from build123d import *

# Parameters (mm, degrees)
SKETCH1_R              = 13.768224287
SKETCH1_R_2            = 12.268224287
SKETCH1_R_3            = 10.768224287
BOSS_EXTRUDE1_DEPTH    = 6.5
CUT_EXTRUDE3_DEPTH     = 519.353793234
CUT_EXTRUDE1_START     = -1.3
CUT_EXTRUDE1_DEPTH     = 13
CUT_EXTRUDE8_START     = -1.75
CUT_EXTRUDE8_OUTLINE_R = 10.768224287
CUT_EXTRUDE8_DEPTH     = 1.75
SKETCH6_R              = 12.268224287
CUT_EXTRUDE9_DEPTH     = 1.3
CUT_EXTRUDE12_START    = -1.75
CUT_EXTRUDE12_DEPTH    = 1.75
SKETCH8_R              = 2.5
CUT_EXTRUDE13_DEPTH    = 63.803249571
CHAMFER1_SIZE          = 2.5
CUT_EXTRUDE14_START    = -3.45
CUT_EXTRUDE14_DEPTH    = 3.45


# Read off the part's stored shape, not the designer's step: Cut-Extrude8
with BuildPart() as part:
    # Sketch1 → Boss-Extrude1 (new, symmetric)
    # profile 1 of 6: a face of its own
    with BuildSketch(Plane(origin=(0, 0, 0), x_dir=(0, 0, -1), z_dir=(1, 0, 0))):
        with BuildLine():
            Line((0, 5), (0, 0))
            Line((0, 0), (15, 0))
            Line((15, 0), (15, 0.231775713))
            Line((15, 0.231775713), (15.418491318, 8.357342638))
            ThreePointArc((15.418491318, 8.357342638), (14.445072398, 11.461887277), (14.227329557, 14.708166664))
            Line((14.227329557, 14.708166664), (13.727329557, 5))
            Line((13.727329557, 5), (0, 5))
        make_face()
    # profile 2 of 6: a face of its own
    with BuildSketch(Plane(origin=(0, 0, 0), x_dir=(0, 0, -1), z_dir=(1, 0, 0))):
        with BuildLine():
            Line((15.418491318, 8.357342638), (15, 0.231775713))
            Line((15, 0.231775713), (27.977329557, 0.231775713))
            ThreePointArc((27.977329557, 0.231775713), (20.498204345, 2.440299049), (15.418491318, 8.357342638))
        make_face()
    # profile 3 of 6: a face of its own
    with BuildSketch(Plane(origin=(0, 0, 0), x_dir=(0, 0, -1), z_dir=(1, 0, 0))):
        with BuildLine():
            ThreePointArc((40.536167797, 8.357342638), (35.45645477, 2.440299049), (27.977329557, 0.231775713))
            Line((27.977329557, 0.231775713), (40.954659115, 0.231775713))
            Line((40.954659115, 0.231775713), (40.536167797, 8.357342638))
        make_face()
    # profile 4 of 6: a face of its own
    with BuildSketch(Plane(origin=(0, 0, 0), x_dir=(0, 0, -1), z_dir=(1, 0, 0))):
        with BuildLine():
            Line((42.227329557, 5), (41.727329557, 14.708166664))
            ThreePointArc((41.727329557, 14.708166664), (41.740997019, 14.354200561), (41.745553845, 14))
            ThreePointArc((41.745553845, 14), (41.439812643, 11.114597224), (40.536167797, 8.357342638))
            Line((40.536167797, 8.357342638), (40.954659115, 0.231775713))
            Line((40.954659115, 0.231775713), (40.954659115, 0))
            Line((40.954659115, 0), (55.954659115, 0))
            Line((55.954659115, 0), (55.954659115, 5))
            Line((55.954659115, 5), (42.227329557, 5))
        make_face()
    # profile 5 of 6: a face of its own
    with BuildSketch(Plane(origin=(0, 0, 0), x_dir=(0, 0, -1), z_dir=(1, 0, 0))):
        with Locations((27.977329557, 14)):
            Circle(SKETCH1_R)
        with Locations((27.977329557, 14)):
            Circle(SKETCH1_R_2, mode=Mode.SUBTRACT)
    # profile 6 of 6: a face of its own
    with BuildSketch(Plane(origin=(0, 0, 0), x_dir=(0, 0, -1), z_dir=(1, 0, 0))):
        with Locations((27.977329557, 14)):
            Circle(SKETCH1_R_2)
        with Locations(Location((27.977329557, 14, 0), (0, 0, 180))):
            Circle(SKETCH1_R_3, mode=Mode.SUBTRACT)
    extrude(amount=BOSS_EXTRUDE1_DEPTH, both=True)

    # Sketch3 → Cut-Extrude3 (cut, through all)
    with BuildSketch(Plane(origin=(0, -487.515659686, 0), x_dir=(-1, 0, 0), z_dir=(0, 0, 1))):
        Polygon((-4.75, -502.22382635), (-6.5, -492.515659686), (-6.5, -515.283883974), (-4.75, -515.283883974), align=None)
        Polygon((6.5, -515.283883974), (6.5, -492.515659686), (4.75, -502.22382635), (4.75, -515.283883974), align=None)
    extrude(amount=-CUT_EXTRUDE3_DEPTH, mode=Mode.SUBTRACT)

    # Sketch2 → Cut-Extrude1 (cut)
    with BuildSketch(Plane(origin=(0, 0, 0), x_dir=(0, 0, -1), z_dir=(1, 0, 0)).offset(CUT_EXTRUDE1_START)):
        with BuildLine():
            Line((15, 0.231775713), (27.977329557, 0.231775713))
            ThreePointArc((27.977329557, 0.231775713), (20.498204345, 2.440299049), (15.418491318, 8.357342638))
            Line((15.418491318, 8.357342638), (15, 0.231775713))
        make_face()
        with BuildLine():
            Line((27.977329557, 0.231775713), (40.954659115, 0.231775713))
            Line((40.954659115, 0.231775713), (40.536167797, 8.357342638))
            ThreePointArc((40.536167797, 8.357342638), (35.45645477, 2.440299049), (27.977329557, 0.231775713))
        make_face()
    cut_extrude1 = extrude(amount=-CUT_EXTRUDE1_DEPTH, mode=Mode.SUBTRACT)

    # Cut-Extrude8 outline → Cut-Extrude8 (cut)
    with BuildSketch(Plane.ZY.offset(6.5).offset(CUT_EXTRUDE8_START)):
        with BuildLine():
            Line((-40.225097809, 14.708166664), (-40.536167797, 8.357342638))
            ThreePointArc((-40.536167797, 8.357342638), (-27.977329557, 0.231775713), (-15.418491318, 8.357342638))
            Line((-15.418491318, 8.357342638), (-15.729561306, 14.708166664))
            ThreePointArc((-15.729561306, 14.708166664), (-27.977329557, 26.268224287), (-40.225097809, 14.708166664))
        make_face()
        with Locations((-27.977329557, 14)):
            Circle(CUT_EXTRUDE8_OUTLINE_R, mode=Mode.SUBTRACT)
    extrude(amount=CUT_EXTRUDE8_DEPTH, mode=Mode.SUBTRACT)

    # Sketch6 → Cut-Extrude9 (cut)
    with BuildSketch(Plane.ZY.offset(4.75)):
        with Locations(Location((-27.977329557, 14, 0), (0, 0, 270))):
            Circle(SKETCH6_R)
    cut_extrude9 = extrude(amount=-CUT_EXTRUDE9_DEPTH, mode=Mode.SUBTRACT)

    # Mirror2: Cut-Extrude1, Cut-Extrude9 across plane
    add(cut_extrude1.mirror(Plane(origin=(0, 0, 0), x_dir=(0, 0, 1), z_dir=(1, 0, 0))), mode=Mode.SUBTRACT)
    add(cut_extrude9.mirror(Plane(origin=(0, 0, 0), x_dir=(0, 0, 1), z_dir=(1, 0, 0))), mode=Mode.SUBTRACT)

    # Sketch7 → Cut-Extrude12 (cut)
    with BuildSketch(Plane(origin=(6.5, 0, 0), x_dir=(0, 0, -1), z_dir=(1, 0, 0)).offset(CUT_EXTRUDE12_START)):
        with BuildLine():
            ThreePointArc((38.396734532, 5), (39.588438578, 6.600936051), (40.536167797, 8.357342638))
            Line((40.536167797, 8.357342638), (40.225097809, 14.708166664))
            ThreePointArc((40.225097809, 14.708166664), (27.977329557, 26.268224287), (15.729561306, 14.708166664))
            Line((15.729561306, 14.708166664), (15.418491318, 8.357342638))
            ThreePointArc((15.418491318, 8.357342638), (16.366220536, 6.600936051), (17.557924583, 5))
            Line((17.557924583, 5), (22.065083427, 5))
            ThreePointArc((22.065083427, 5), (27.977329557, 3.231775713), (33.889575687, 5))
            Line((33.889575687, 5), (38.396734532, 5))
        make_face()
        with BuildLine():
            Line((22.065083427, 5), (17.557924583, 5))
            ThreePointArc((17.557924583, 5), (27.977329557, 0.231775713), (38.396734532, 5))
            Line((38.396734532, 5), (33.889575687, 5))
            ThreePointArc((33.889575687, 5), (27.977329557, 3.231775713), (22.065083427, 5))
        make_face()
    extrude(amount=CUT_EXTRUDE12_DEPTH, mode=Mode.SUBTRACT)

    # Sketch8 → Cut-Extrude13 (cut, through all)
    with BuildSketch(Plane.XZ):
        with Locations(Location((0, -48.977329557, 0), (0, 0, 270))):
            Circle(SKETCH8_R)
        with Locations(Location((0, -6.977329557, 0), (0, 0, 270))):
            Circle(SKETCH8_R)
    extrude(amount=-CUT_EXTRUDE13_DEPTH, mode=Mode.SUBTRACT)

    # Chamfer1
    chamfer1_edges = [part.edges().sort_by_distance(p)[0] for p in [
        (-6.5, 2.5, 0),
        (6.5, 2.5, -55.954659115),
        (-6.5, 2.5, -55.954659115),
        (6.5, 2.5, 0),
    ]]
    chamfer(chamfer1_edges, length=CHAMFER1_SIZE)

    # Sketch9 → Cut-Extrude14 (cut)
    with BuildSketch(Plane.ZY.offset(3.45).offset(CUT_EXTRUDE14_START)):
        with BuildLine():
            Line((-38.451328521, 16.5), (-39.988129995, 16.5))
            ThreePointArc((-39.988129995, 16.5), (-40.245553845, 14), (-39.988129995, 11.5))
            Line((-39.988129995, 11.5), (-38.451328521, 11.5))
            ThreePointArc((-38.451328521, 11.5), (-38.745553845, 14), (-38.451328521, 16.5))
        make_face()
        with BuildLine():
            ThreePointArc((-15.70910527, 14), (-15.773630921, 15.256609231), (-15.966529119, 16.5))
            Line((-15.966529119, 16.5), (-17.503330593, 16.5))
            ThreePointArc((-17.503330593, 16.5), (-17.282914559, 15.258627083), (-17.20910527, 14))
            ThreePointArc((-17.20910527, 14), (-17.282914559, 12.741372917), (-17.503330593, 11.5))
            Line((-17.503330593, 11.5), (-15.966529119, 11.5))
            ThreePointArc((-15.966529119, 11.5), (-15.773630921, 12.743390769), (-15.70910527, 14))
        make_face()
    extrude(amount=CUT_EXTRUDE14_DEPTH, mode=Mode.SUBTRACT)


solid = part.part
The listing builds one solid part. Answer for the finished solid, in the listing's coordinates (mm). A direction names the side the tool comes from. Round coordinates to 2 decimals unless told otherwise and drop trailing zeros. Write each loop counter-clockwise with the first axis right and the second up, starting at its lowest first coordinate (ties: lowest second). Pieces come first, ordered by that corner, then holes. Notation, with made-up numbers: M 26.25,29 L 46.25,29 A32 cw 46.25,57 Z; hole C 39,-6 d2. An arc over 180 degrees is marked long. Write each question's results on one line, items separated by ' | '. Start each with the question number.
Item 1: Find section A-A on z = -35. Write down the section's boundary in (x, y).
Item 2: The mould has two halves that part along Y. Classify faces 4 (the flat face through (-2, 16.5, -17)), 5 (the flat face through (6.5, 3, -9)), 6 (the flat face through (-5.06, 10.166, -40.448)): +Y half, -Y half, draft (parallel to the pull), parting line (faces both ways), or undercut.
Item 3: Find section C-C on z = -12. Write down the section's boundary in (x, y).
Item 4: Given pin 1 Ø2 at (x, z) = (2, -39.5) entering from -Y; pin 2 Ø4.5 at (y, z) = (4, -31) entering from -X; pin 3 Ø1.7 at (x, z) = (-2.5, -39) entering from +Y, each flat-ended and moving along its own axis, determine where each tip first touches the part or whether it passes through.
Item 5: Straight lines are drawn through the part: probe 1 along X at (y, z) = (2.75, -31); probe 2 along Y at (x, z) = (0.25, -46); probe 3 along X at (y, z) = (5, -17.5). For each, find the intervals that lie inside material, in ascending order.
Item 6: Which of the six approach directions +Z, -Z, +X, -X, +Y, -Y give full straight-line access (tool end or side, diameter ignored) to faces 1 (the flat face through (-5.187, 10.783, -15.537)), 2 (the flat face through (0, 0.232, -28)), 3 (the flat face through (0, 5, -10))?
Item 7: Find section B-B on y = 25.75. Write down the section's boundary in (x, z), and give its area (3 significant figures).
Answer block:
1) outline: M -4.75,2.16 L -1.3,2.16 L -1.3,0.23 L 1.3,0.23 L 1.3,2.16 L 4.75,2.16 L 4.75,3.94 L 3.45,3.94 L 3.45,5.84 L -3.45,5.84 L -3.45,3.94 L -4.75,3.94 Z; M -4.75,24.06 L -3.45,24.06 L -3.45,22.16 L 3.45,22.16 L 3.45,24.06 L 4.75,24.06 L 4.75,25.84 L -4.75,25.84 Z
2) face 4: undercut | face 5: draft | face 6: -Y half
3) outline: M -6.5,0 L 6.5,0 L 6.5,5 L -6.5,5 Z
4) pin 1: stops at y = 0.23 | pin 2: stops at x = -4.75 | pin 3: stops at y = 23.28
5) probe 1: x = -3.45 to 3.45 | probe 2: y = 0 to 5 | probe 3: x = -1.3 to 1.3
6) face 1: -X, -Y | face 2: +X, -X, -Y | face 3: +Z, +X, -X, +Y
7) outline: M -4.75,-35.15 L 4.75,-35.15 L 4.75,-31.51 L 3.45,-31.51 L 3.45,-24.45 L 4.75,-24.45 L 4.75,-20.8 L -4.75,-20.8 L -4.75,-24.45 L -3.45,-24.45 L -3.45,-31.51 L -4.75,-31.51 Z | area: 118 mm²
